Autodesk Inventor part; units mm, degrees
ref_plane "YZ Plane" through (0, 0, 0) normal (1, 0, 0) x (0, 1, 0)
ref_plane "XZ Plane" through (0, 0, 0) normal (0, 1, 0) x (-1, 0, 0)
ref_plane "XY Plane" through (0, 0, 0) normal (0, 0, 1) x (1, 0, 0)
sketch "Skizze1" plane through (0, 0, 0) normal (0, 1, 0) x (-1, 0, 0)
  line L0 (6.1, 0) -> (8.6, 0.5101)
  arc A0 (8.6, 0.5101) -> (9, 1) centre (8.5, 1) ccw
  line L1 (9, 1) -> (6.8, 1)
  line L2 (6.8, 1) -> (6.8, 5)
  line L3 (6.8, 5) -> (5.1, 5)
  line L4 (5.1, 5) -> (5.1, 0)
  line L5 (5.1, 0) -> (6.1, 0)
  line L6 (0, 0) -> (0, 11) construction
  dimension "d0" = 6.8
  dimension "d1" = 5.1
  dimension "d2" = 1
  dimension "d3" = 9
  dimension "d4" = 1
  dimension "d6" = 4
  dimension "d8" = 0.5
revolve "Umdrehung1" add sketch "Skizze1" angle 360 about axis through (0, 0, 0) along (0, 0, 1)
properties part number "08-02-01-010_buttonSide" material "ABS-Kunststoff(1)"
Build history of the part. All positions in model axes, mm. A direction names the side the tool comes from. Round coordinates to 2 decimals unless told otherwise and drop trailing zeros. Loops run counter-clockwise (first coordinate to the right, second up) from the corner with the lowest first, then second, coordinate; pieces in that order, holes last.
Item 1: Drill centre lines: line 1 along X through (y, z) = (0, 1.5); line 2 along X through (y, z) = (3.25, 4). Where is each one in solid material? Low to high.
Item 2: Which spindle directions (+Z, -Z, +X, -X, +Y, -Y) get a long thin tool onto all of the face, cutting with end or side? Do faces 1 (the face through (-2, -5, 5)), 2 (the face through (-1, -7, 1)). Say none if no direction does.
Item 3: Saw through at A-A (y = 0). List the corners of the cut face in (x, z), then the cut area to 3 significant figures.
Item 4: Two-plate mould, pull along Y, no slides. Class faces 3 (the face through (-2.4, -4.5, 2.5)), 4 (the face through (4, 4, 0)), 5 (the face through (1.47, 6.64, 3.03)): released by +Y, released by -Y, zero draft, split by the parting line, or undercut.
Item 5: Saw through at C-C (z = 2.8). List the corners of the cut face in (x, y), then the cut area to 3 significant figures.
Item 6: Pin check, flat tips, straight feed: P1, Ø2, axis at x = 5.5, y = 7, coming from the -Z side; P2, Ø1.5, axis at x = 4, z = 1.5, coming from the +Y side; P3, Ø3, axis at y = -1.5, z = 4, coming from the +X side. Stop position of each tip, or through.
Worked answers:
1. line 1: x = -6.8 to -5.1, 5.1 to 6.8
1. line 2: x = -5.97 to -3.93, 3.93 to 5.97
2. face 1: +Z, +X, -X, +Y, -Y
2. face 2: +Z
3. outline: (-9, 1) arc R0.5 ccw to (-8.6, 0.51) - (-6.1, 0) - (-5.1, 0) - (-5.1, 5) - (-6.8, 5) - (-6.8, 1) - close; (5.1, 0) - (6.1, 0) - (8.6, 0.51) arc R0.5 ccw to (9, 1) - (6.8, 1) - (6.8, 5) - (5.1, 5) - close
3. area: 19.6 mm2
4. face 3: undercut
4. face 4: zero draft
4. face 5: split by the parting line
5. outline: circle Ø13.6 at (0, 0); hole circle Ø10.2 at (0, 0)
5. area: 63.6 mm2
6. P1: stops at z = 0.37
6. P2: stops at y = 8.32
6. P3: stops at x = 6.8
